```python
from build123d import *

# Parameters (mm, degrees)
SKETCH_1_W          = 38.1
SKETCH_1_H          = 44
SENSOR_BASE_DEPTH   = 5
PROTECTOR_DEPTH     = 22.2
SKETCH_4_R          = 1.575
CUT_EXTRUDE_1_DEPTH = 37.602493084
SKETCH_5_W          = 38.1
SKETCH_5_H          = 5
EXTRUDE_3_DEPTH     = 29
EXTRUDE_4_DEPTH     = 4
SKETCH_9_W          = 6
SKETCH_9_H          = 29.5
EXTRUDE_5_DEPTH     = 9
SKETCH_10_W         = 17
SKETCH_10_H         = 10
EXTRUDE_6_DEPTH     = 9
FILLET_2_R          = 4
FILLET_3_R          = 4
FILLET_4_R          = 4
FILLET_5_R          = 4
FILLET_6_R          = 4
CUT_EXTRUDE_6_REACH = 83.936
SKETCH_26_R         = 2.1
SKETCH_30_W         = 14.05
SKETCH_30_H         = 8
CUT_EXTRUDE_7_DEPTH = 5
CUT_EXTRUDE_8_REACH = 75.991
SKETCH_31_R         = 1.575
FILLET_7_R          = 1
FILLET_8_R          = 1
FILLET_9_R          = 1


with BuildPart() as part:
    # 草图1 → Sensor_base (new body)
    with BuildSketch(Plane(origin=(0, 0, 0), x_dir=(1, 0, 0), z_dir=(0, 1, 0))):
        Rectangle(SKETCH_1_W, SKETCH_1_H)
    extrude(amount=SENSOR_BASE_DEPTH)

    # 草图2 → Protector (add)
    with BuildSketch(Plane(origin=(0, 5, 0), x_dir=(1, 0, 0), z_dir=(0, 1, 0))):
        Polygon((-19.05, 22), (-19.05, -19.5), (-16.05, -19.5), (-16.05, 19), (16.05, 19), (16.05, -19.5), (19.05, -19.5), (19.05, 18), (19.05, 22), align=None)
    extrude(amount=PROTECTOR_DEPTH)

    # 草图4 → 切除-拉伸1 (cut, through all)
    with BuildSketch(Plane(origin=(0, 5, 0), x_dir=(1, 0, 0), z_dir=(0, 1, 0))):
        with Locations(Location((0, 13, 0), (0, 0, 270))):
            Circle(SKETCH_4_R)
        with Locations(Location((-10, 3, 0), (0, 0, 270))):
            Circle(SKETCH_4_R)
        with Locations(Location((10, 3, 0), (0, 0, 270))):
            Circle(SKETCH_4_R)
        with Locations(Location((0, -7, 0), (0, 0, 270))):
            Circle(SKETCH_4_R)
    extrude(amount=-CUT_EXTRUDE_1_DEPTH, mode=Mode.SUBTRACT)

    # 草图5 → 凸台-拉伸3 (add)
    with BuildSketch(Plane.XY.offset(22)):
        with Locations((0, 2.5)):
            Rectangle(SKETCH_5_W, SKETCH_5_H)
    extrude(amount=EXTRUDE_3_DEPTH)

    # 草图8 → 凸台-拉伸4 (add)
    with BuildSketch(Plane.XY.offset(51)):
        Polygon((0, 0), (-27.9, 0), (-27.9, 29.5), (27.9, 29.5), (27.9, 0), align=None)
    extrude(amount=EXTRUDE_4_DEPTH)

    # 草图9 → 凸台-拉伸5 (add)
    with BuildSketch(Plane.XY.offset(55)):
        with Locations((-10.9, 14.75)):
            Rectangle(SKETCH_9_W, SKETCH_9_H)
    extrude(amount=EXTRUDE_5_DEPTH)

    # 草图10 → 凸台-拉伸6 (add)
    with BuildSketch(Plane.XY.offset(55)):
        with Locations((19.4, 24.5)):
            Rectangle(SKETCH_10_W, SKETCH_10_H)
        with Locations((19.4, 5)):
            Rectangle(SKETCH_10_W, SKETCH_10_H)
    extrude(amount=EXTRUDE_6_DEPTH)

    # 圆角2
    fillet_2_edges = [part.edges().sort_by_distance(p)[0] for p in [
        (19.4, 29.5, 64),
    ]]
    fillet(fillet_2_edges, radius=FILLET_2_R)

    # 圆角3
    fillet_3_edges = [part.edges().sort_by_distance(p)[0] for p in [
        (19.4, 19.5, 64),
    ]]
    fillet(fillet_3_edges, radius=FILLET_3_R)

    # 圆角4
    fillet_4_edges = [part.edges().sort_by_distance(p)[0] for p in [
        (19.4, 0, 64),
        (19.4, 10, 64),
    ]]
    fillet(fillet_4_edges, radius=FILLET_4_R)

    # 圆角5
    fillet_5_edges = [part.edges().sort_by_distance(p)[0] for p in [
        (-10.9, 0, 64),
        (-10.9, 29.5, 64),
    ]]
    fillet(fillet_5_edges, radius=FILLET_5_R)

    # 圆角6
    fillet_6_edges = [part.edges().sort_by_distance(p)[0] for p in [
        (-17.55, 27.2, 19.5),
        (17.55, 27.2, 19.5),
    ]]
    fillet(fillet_6_edges, radius=FILLET_6_R)

    # 草图26 → 切除-拉伸6 (cut, up to next)
    with BuildSketch(Plane.ZY.offset(13.9), mode=Mode.PRIVATE) as cut_extrude_6_sk1:
        with Locations(Location((59.5, 5, 0), (0, 0, 270))):
            Circle(SKETCH_26_R)
    cut_extrude_6_tool1 = extrude(cut_extrude_6_sk1.sketch, amount=-CUT_EXTRUDE_6_REACH, mode=Mode.PRIVATE) & part.part
    # 草图26 → 切除-拉伸6 (cut, up to next)
    with BuildSketch(Plane.ZY.offset(13.9), mode=Mode.PRIVATE) as cut_extrude_6_sk2:
        with Locations(Location((59.5, 15, 0), (0, 0, 270))):
            Circle(SKETCH_26_R)
    cut_extrude_6_tool2 = extrude(cut_extrude_6_sk2.sketch, amount=-CUT_EXTRUDE_6_REACH, mode=Mode.PRIVATE) & part.part
    # 草图26 → 切除-拉伸6 (cut, up to next)
    with BuildSketch(Plane.ZY.offset(13.9), mode=Mode.PRIVATE) as cut_extrude_6_sk3:
        with Locations(Location((59.5, 25, 0), (0, 0, 270))):
            Circle(SKETCH_26_R)
    cut_extrude_6_tool3 = extrude(cut_extrude_6_sk3.sketch, amount=-CUT_EXTRUDE_6_REACH, mode=Mode.PRIVATE) & part.part
    add(cut_extrude_6_tool1.solids().sort_by_distance((-13.9, 5, 59.5))[0], mode=Mode.SUBTRACT)
    add(cut_extrude_6_tool2.solids().sort_by_distance((-13.9, 15, 59.5))[0], mode=Mode.SUBTRACT)
    add(cut_extrude_6_tool3.solids().sort_by_distance((-13.9, 25, 59.5))[0], mode=Mode.SUBTRACT)

    # 草图30 → 切除-拉伸7 (cut)
    with BuildSketch(Plane(origin=(0, 5, 0), x_dir=(1, 0, 0), z_dir=(0, 1, 0))):
        Polygon((0, -44), (5, -44), (5, -36), (-5, -36), (-5, -44), align=None)
        with Locations((12.025, -40)):
            Rectangle(SKETCH_30_W, SKETCH_30_H)
    extrude(amount=-CUT_EXTRUDE_7_DEPTH, mode=Mode.SUBTRACT)

    # 草图31 → 切除-拉伸8 (cut, up to next)
    with BuildSketch(Plane(origin=(0, 5, 0), x_dir=(1, 0, 0), z_dir=(0, 1, 0)), mode=Mode.PRIVATE) as cut_extrude_8_sk1:
        with Locations(Location((12.025, -32.5, 0), (0, 0, 270))):
            Circle(SKETCH_31_R)
    cut_extrude_8_tool1 = extrude(cut_extrude_8_sk1.sketch, amount=-CUT_EXTRUDE_8_REACH, mode=Mode.PRIVATE) & part.part
    # 草图31 → 切除-拉伸8 (cut, up to next)
    with BuildSketch(Plane(origin=(0, 5, 0), x_dir=(1, 0, 0), z_dir=(0, 1, 0)), mode=Mode.PRIVATE) as cut_extrude_8_sk2:
        with Locations(Location((12.025, -47.5, 0), (0, 0, 270))):
            Circle(SKETCH_31_R)
    cut_extrude_8_tool2 = extrude(cut_extrude_8_sk2.sketch, amount=-CUT_EXTRUDE_8_REACH, mode=Mode.PRIVATE) & part.part
    add(cut_extrude_8_tool1.solids().sort_by_distance((12.025, 5, 32.5))[0], mode=Mode.SUBTRACT)
    add(cut_extrude_8_tool2.solids().sort_by_distance((12.025, 5, 47.5))[0], mode=Mode.SUBTRACT)

    # 圆角7
    fillet_7_edges = [part.edges().sort_by_distance(p)[0] for p in [
        (19.05, 13.6, -22),
    ]]
    fillet(fillet_7_edges, radius=FILLET_7_R)

    # 圆角8
    fillet_8_edges = [part.edges().sort_by_distance(p)[0] for p in [
        (19.05, 0, 7.5),
        (-0.5, 0, -22),
        (18.757106781, 0, -21.707106781),
        (-19.05, 0, 14.5),
        (-19.05, 13.6, -22),
    ]]
    fillet(fillet_8_edges, radius=FILLET_8_R)

    # 圆角9
    fillet_9_edges = [part.edges().sort_by_distance(p)[0] for p in [
        (-16.05, 27.2, -1.75),
        (19.05, 27.2, -2.75),
        (-16.05, 14.1, 19.5),
        (-16.05, 26.028427125, 18.328427125),
        (-19.05, 14.1, 19.5),
        (-19.05, 26.028427125, 18.328427125),
        (19.05, 14.1, 19.5),
        (19.05, 26.028427125, 18.328427125),
        (16.05, 14.1, 19.5),
        (16.05, 26.028427125, 18.328427125),
        (0, 27.2, -19),
        (16.05, 27.2, -1.75),
        (0, 27.2, -22),
        (18.757106781, 27.2, -21.707106781),
        (-19.05, 27.2, -2.75),
        (-18.757106781, 27.2, -21.707106781),
    ]]
    fillet(fillet_9_edges, radius=FILLET_9_R)


solid = part.part
```
For this review, take the finished solid that the model builds, in its own axes (mm). A direction names the side the tool comes from. Coordinates: 2 decimals unless noted, no trailing zeros. Write each loop counter-clockwise with the first axis right and the second up, starting at its lowest first coordinate (ties: lowest second). Pieces come first, ordered by that corner, then holes.
(1) Add section C-C on y = 15. Give the boundary of the cut face in (x, z).
(2) Wall thickness on probe 1 along X at (y, z) = (3.45, -3) (3 decimals); probe 2 along X at (y, z) = (3.45, 32.5); probe 3 along Z at (x, y) = (10.5, 17.25): over which ranges is each line inside the solid? List them lowest first.
(3) Add section D-D on x = 21. Give the boundary of the cut face in (y, z).
(4) The part is to be moulded in two halves that separate along Z. For faces 1 (the face through (19.05, 2, 47)), 2 (the face through (-5, 3, 40)), 3 (the face through (19, 25, 64)), say which applies: +Z half, -Z half, draft (parallel to the pull), parting line (faces both ways), or undercut.
(5) Add section B-B on x = 0. Give the boundary of the cut face in (y, z) (3 decimals), then the cut area to 3 significant figures.
(6) Tool access review of faces 4 (the face through (-17.543, 25.997, 18.359)), 5 (the face through (-19.05, 13, -2)), 6 (the face through (7, 3, 36)), 7 (the face through (-7.9, 15, 57)), 8 (the face through (19, 19.5, 57)): name each direction out of +Z, -Z, +X, -X, +Y, -Y from which nothing blocks a thin tool from reaching the whole face with its end or side.
(7) Add section A-A on z = 32.5. Give the boundary of the cut face in (x, y).
(8) For pin 1 Ø2.5 at (y, z) = (3.5, 49) entering from +X; pin 2 Ø11 at (x, z) = (-5.5, -4) entering from +Y; pin 3 Ø4 at (y, z) = (15, 59.5) entering from -X; pin 4 Ø3 at (x, y) = (9, 26) entering from +Z, all flat-tipped, find the tip position at first contact; note any pin that passes through.
Answer sheet:
1. outline: (-27.9, 51) - (27.9, 51) - (27.9, 55) - (-7.9, 55) - (-7.9, 57.4) - (-13.9, 57.4) - (-13.9, 55) - (-27.9, 55) - close; (-19.05, -21) arc R1 ccw to (-18.05, -22) - (18.05, -22) arc R1 ccw to (19.05, -21) - (19.05, 18.5) arc R1 ccw to (18.05, 19.5) - (17.05, 19.5) arc R1 ccw to (16.05, 18.5) - (16.05, -19) - (-16.05, -19) - (-16.05, 18.5) arc R1 ccw to (-17.05, 19.5) - (-18.05, 19.5) arc R1 ccw to (-19.05, 18.5) - close; (-13.9, 61.6) - (-7.9, 61.6) - (-7.9, 64) - (-13.9, 64) - close
2. probe 1: x = -19.05 to -11.575, -8.425 to 8.425, 11.575 to 19.05
2. probe 2: x = -19.05 to 10.45, 13.6 to 19.05
2. probe 3: z = -22 to -19, 51 to 55
3. outline: (0, 51) - (29.5, 51) - (29.5, 60) arc R4 ccw to (25.5, 64) - (23.5, 64) arc R4 ccw to (19.5, 60) - (19.5, 55) - (10, 55) - (10, 60) arc R4 ccw to (6, 64) - (4, 64) arc R4 ccw to (0, 60) - close
4. face 1: draft
4. face 2: undercut
4. face 3: +Z half
5. outline: (0, -21) arc R1 ccw to (1, -22) - (26.2, -22) arc R1 ccw to (27.2, -21) - (27.2, -20) arc R1 ccw to (26.2, -19) - (5, -19) - (5, -14.575) - (0, -14.575) - close; (0, -11.425) - (5, -11.425) - (5, 5.425) - (0, 5.425) - close; (0, 8.575) - (5, 8.575) - (5, 36) - (0, 36) - close; (0, 44) - (5, 44) - (5, 51) - (29.5, 51) - (29.5, 55) - (0, 55) - close
5. area: 477 mm2
6. face 4: +X, -X, +Y
6. face 5: -Z, -X, +Y, -Y
6. face 6: +X, +Y, -Y
6. face 7: +Z, +Y, -Y
6. face 8: +Z, +X
7. outline: (-19.05, 1) arc R1 ccw to (-18.05, 0) - (10.45, 0) - (10.45, 5) - (-19.05, 5) - close; (13.6, 0) - (18.05, 0) arc R1 ccw to (19.05, 1) - (19.05, 5) - (13.6, 5) - close
8. pin 1: stops at x = 19.05
8. pin 2: stops at y = 5
8. pin 3: passes through
8. pin 4: stops at z = 55
